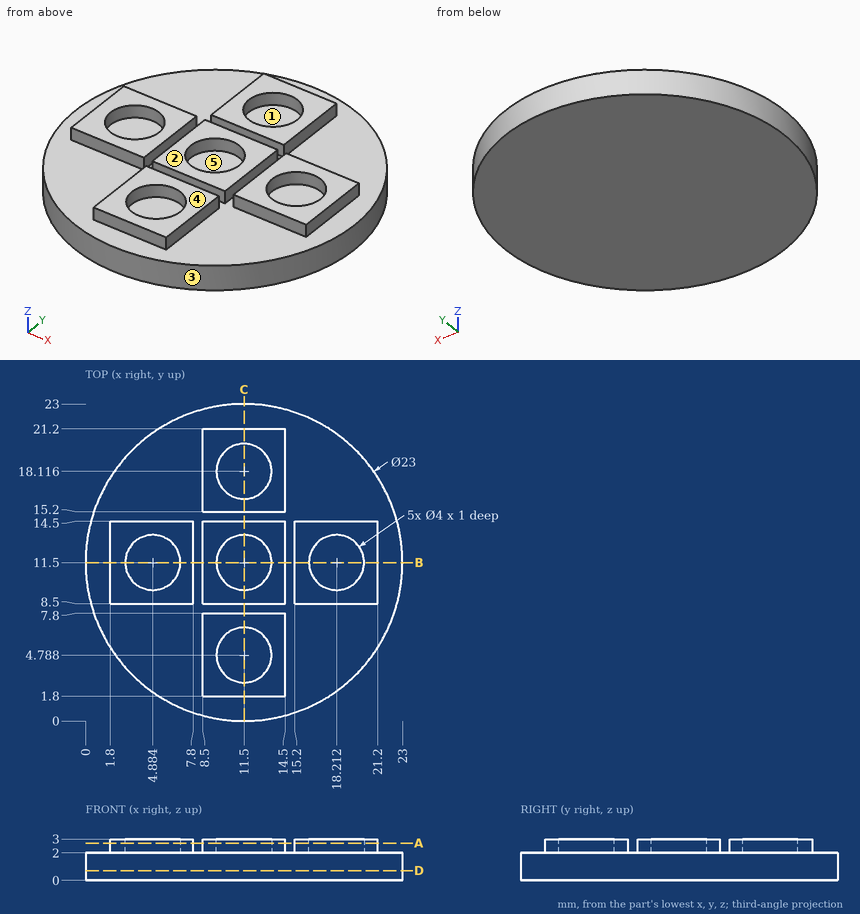
Design review of the part shown in the three views and the two pictorial views. Dimensions are in mm from the part's minimum x, y and z. A direction names the side the tool comes from. Coordinates: 2 decimals unless noted, no trailing zeros. Order: outer loops, then holes, each group sorted by start corner. A loop starts at its lowest first (then second) coordinate and runs counter-clockwise, first axis right, second up.
1) Take a section at B-B, the plane y = 11.5. Give the boundary of the cut face in (x, z) (1 decimal).
2) Take a section at A-A, the plane z = 2.7. State how many separate pieces and enclosed holes the cut face has, and give its area (3 significant figures).
3) For the marked faces 1 and 2, list the 3-axis set-ups (+Z, -Z, +X, -X, +Y, -Y) from which the entire face can be reached by the end or side of a thin tool; tool diameter is ignored.
4) Wall thickness on line 1 along Y through (x, z) = (11.5, 2.45) (1 decimal); line 2 along X through (y, z) = (9, 2.6): over which ranges is each line inside the solid? List them lowest first.
5) Take a section at D-D, the plane z = 0.7. Give the boundary of the cut face in (x, y).
6) Clearance check with flat-ended pins moving along their axes: pin 1 (1.2 mm diameter, centred on x = 6, y = 11, fed in from +Z); pin 2 (10 mm diameter, centred on x = 15, y = 8, fed in from +Z); pin 3 (1 mm diameter, centred on y = 7, z = 1.5, fed in from +X); pin 4 (0.5 mm diameter, centred on y = 6, z = 2.5, fed in from +X). State where each tip first meets the part, or that it passes through.
7) Mouldability with a two-part tool opening along Y and no side actions: class the marked faces 3, 4 and 5 as +Y half, -Y half, draft (parallel to the pull), parting line (faces both ways), or undercut.
8) Take a section at C-C, the plane x = 11.5. Give the boundary of the cut face in (y, z) (1 decimal).
Returned:
1. outline: (0, 0) - (23, 0) - (23, 2) - (21.2, 2) - (21.2, 3) - (20.2, 3) - (20.2, 2) - (16.2, 2) - (16.2, 3) - (15.2, 3) - (15.2, 2) - (14.5, 2) - (14.5, 3) - (13.5, 3) - (13.5, 2) - (9.5, 2) - (9.5, 3) - (8.5, 3) - (8.5, 2) - (7.8, 2) - (7.8, 3) - (6.9, 3) - (6.9, 2) - (2.9, 2) - (2.9, 3) - (1.8, 3) - (1.8, 2) - (0, 2) - close
2. separate pieces: 5
2. enclosed holes: 5
2. area: 117 mm2
3. face 1: +Z
3. face 2: +Z, +X, -X, +Y, -Y
4. line 1: y = 1.8 to 2.8, 6.8 to 7.8, 8.5 to 9.5, 13.5 to 14.5, 15.2 to 16.1, 20.1 to 21.2
4. line 2: x = 1.8 to 7.8, 8.5 to 14.5, 15.2 to 21.2
5. outline: circle Ø23 at (11.5, 11.5)
6. pin 1: stops at z = 2
6. pin 2: stops at z = 3
6. pin 3: stops at x = 22.28
6. pin 4: stops at x = 14.5
7. face 3: parting line
7. face 4: draft
7. face 5: undercut
8. outline: (0, 0) - (23, 0) - (23, 2) - (21.2, 2) - (21.2, 3) - (20.1, 3) - (20.1, 2) - (16.1, 2) - (16.1, 3) - (15.2, 3) - (15.2, 2) - (14.5, 2) - (14.5, 3) - (13.5, 3) - (13.5, 2) - (9.5, 2) - (9.5, 3) - (8.5, 3) - (8.5, 2) - (7.8, 2) - (7.8, 3) - (6.8, 3) - (6.8, 2) - (2.8, 2) - (2.8, 3) - (1.8, 3) - (1.8, 2) - (0, 2) - close
